Model file for the job. Use its own axes, mm. Give positions to 0.01 mm unless a question says otherwise; leave off trailing zeros. Loops run counter-clockwise (first coordinate to the right, second up) from the corner with the lowest first, then second, coordinate; pieces in that order, holes last. Notation, with made-up numbers: M -17,-24.75 L 22,-24.75 A17 cw 22,-16.75 Z; hole C 14.5,5 d9. An arc over 180 degrees is marked long. Answer in a Markdown table with one row per item.
```python
from build123d import *

# Parameters (mm, degrees)
PAD001_DEPTH      = 2
PAD001_DEPTH_BACK = 2
SKETCH018_W       = 25
SKETCH018_H       = 75
PAD017_DEPTH      = 1


with BuildPart() as body001:
    # Sketch002 → Pad001 (new body, two sides)
    with BuildSketch(Plane.XY) as pad001_sk:
        Polygon((13, 56.25), (6.25, 18.75), (18.75, 18.75), align=None)
    extrude(amount=PAD001_DEPTH)
    extrude(pad001_sk.sketch, amount=-PAD001_DEPTH_BACK)


with BuildPart() as body016:
    # Sketch018 → Pad017 (new body)
    with BuildSketch(Plane.XY):
        with Locations((12.5, 37.5)):
            Rectangle(SKETCH018_W, SKETCH018_H)
    extrude(amount=PAD017_DEPTH)

    # Boolean001: cut Body001
    add(body001.part, mode=Mode.SUBTRACT)


solid = body016.part
```
(1) Wall check: L1, parallel to X at y = 25.5, z = 0.7 (3 decimals); L2, parallel to X at y = 36, z = 0.95 (3 decimals). Give the ranges that are in metal, low to high.
Established:
| item | result |
|---|---|
| L1 | x = 0 to 7.465, 17.715 to 25 |
| L2 | x = 0 to 9.355, 16.105 to 25 |
(2) Saw through at A-A, the plane z = 0.55. Give the cut face in (x, y), and give its area (3 significant figures).
Established:
| item | result |
|---|---|
| outline | M 0,0 L 25,0 L 25,75 L 0,75 Z; hole M 6.25,18.75 L 18.75,18.75 L 13,56.25 Z |
| area | 1,640 mm2 |
(3) Saw through at B-B, the plane x = 15.75. Give the cut face in (y, z).
Established:
| item | result |
|---|---|
| outline | M 0,0 L 18.75,0 L 18.75,1 L 0,1 Z; M 38.32,0 L 75,0 L 75,1 L 38.32,1 Z |
(4) Mould opens along X. For faces 1 (the flat face through (9.67, 37.76, 0.51)), 2 (the flat face through (15.915, 37.238, 0.507)), 3 (the flat face through (9.5, 38, 0)) say: pulls with the +X half, pulls with the -X half, needs draft (parallel to the pull), parting line crosses it, or undercut.
Established:
| item | result |
|---|---|
| face 1 | undercut |
| face 2 | undercut |
| face 3 | needs draft |
(5) Saw through at C-C, the plane y = 26. Give the cut face in (x, z) (3 decimals), and give its area (3 significant figures).
Established:
| item | result |
|---|---|
| outline | M 0,0 L 7.555,0 L 7.555,1 L 0,1 Z; M 17.638,0 L 25,0 L 25,1 L 17.638,1 Z |
| area | 14.9 mm2 |
